Read the model definition and answer for the solid it produces. Units are mm, in the model's axes. A direction names the side the tool comes from. Coordinates: 2 decimals unless noted, no trailing zeros. Loops run counter-clockwise (first coordinate to the right, second up) from the corner with the lowest first, then second, coordinate; pieces in that order, holes last.
Q1. Section D-D (z = -81.5) is taken. Give the vertices of the cut face in (x, y).
Q2. Section C-C (y = -30) is taken. Give the vertices of the cut face in (x, z), then the cut area to 3 significant figures.
Q3. The mould has two halves that part along Y. Classify faces 1 (the face through (0.1, 12.5, -15)), 2 (the face through (0.111, -10.465, 11.056)), 3 (the face through (-0.28, 12.08, -10.12)), 4 (the face through (0, 15, 0)): pulls with the +Y half, pulls with the -Y half, needs draft (parallel to the pull), parting line crosses it, or undercut.
Q4. Which of the six approach directions +Z, -Z, +X, -X, +Y, -Y give full straight-line access (tool end or side, diameter ignored) to faces 5 (the face through (-2.938, -22, -60)), 6 (the face through (0, -27, 7)), 7 (the face through (0.323, -3.605, -35.525))?
Q5. Section A-A (z = -64.5) is taken. Give the vertices of the cut face in (x, y), then the cut area to 3 significant figures.
Q6. Flat-ended cylindrical pins translate along their axes: P1, Ø13, axis at y = -18, z = -64.5, coming from the +X side; P2, Ø3, axis at x = -6, z = -83, coming from the +Y side; P3, Ø4.5, axis at x = 0, y = -35, coming from the +Z side; P4, Ø9, axis at x = 0, z = -10, coming from the -Y side. Find the tip coordinate at first contact, or state that the pin passes through.
Q7. Straight lines are drawn through the part: line 1 (Y direction, x = -1.45, z = -64.5); line 2 (X direction, y = -36, z = -22); line 3 (Z direction, x = -0.75, y = -28). For each, find the intervals that lie inside material, in ascending order.
Q8. Section B-B (z = 0.5) is taken. Give the vertices of the cut face in (x, y), then the cut area to 3 significant figures.
from build123d import *

# Parameters (mm, degrees)
ESBO_O1_R                                            = 7
RESSALTO_EXTRUS_O1_DEPTH                             = 7.9375
ESCAREADO_PARA_PARAFUSO_DE_M_QUINA_COM_C_D           = 5.5
ESCAREADO_PARA_PARAFUSO_DE_M_QUINA_COM_C_DEPTH       = 30
ESCAREADO_PARA_PARAFUSO_DE_M_QUINA_COM_C_CSINK_D     = 10.4
ESCAREADO_PARA_PARAFUSO_DE_M_QUINA_COM_C_CSINK_ANGLE = 90
ESCAREADO_PARA_PARAFUSO_DE_M_QUINA_COM_C_TIP         = 1.652366702
ESCAREADO_PARA_PARAFUSO_DE_M_QUINA_C_2_D             = 6.6
ESCAREADO_PARA_PARAFUSO_DE_M_QUINA_C_2_DEPTH         = 30
ESCAREADO_PARA_PARAFUSO_DE_M_QUINA_C_2_CSINK_D       = 12.6
ESCAREADO_PARA_PARAFUSO_DE_M_QUINA_C_2_CSINK_ANGLE   = 90
ESCAREADO_PARA_PARAFUSO_DE_M_QUINA_C_2_TIP           = 1.982840043
BROCA_DE_ROSQUEAR_PARA_TARRAXA_DE_M5X0_8_D           = 4.2
BROCA_DE_ROSQUEAR_PARA_TARRAXA_DE_M5X0_8_DEPTH       = 20
BROCA_DE_ROSQUEAR_PARA_TARRAXA_DE_M5X0_8_TIP         = 1.2618073
BROCA_DE_ROSQUEAR_PARA_TARRAXA_DE_M5_2_D             = 4.2
BROCA_DE_ROSQUEAR_PARA_TARRAXA_DE_M5_2_DEPTH         = 20
BROCA_DE_ROSQUEAR_PARA_TARRAXA_DE_M5_2_TIP           = 1.2618073
BROCA_DE_ROSQUEAR_PARA_TARRAXA_DE_M6X1_0_D           = 5
BROCA_DE_ROSQUEAR_PARA_TARRAXA_DE_M6X1_0_DEPTH       = 15
BROCA_DE_ROSQUEAR_PARA_TARRAXA_DE_M6X1_0_TIP         = 1.502151548
ESCAREADO_PARA_SFHCS_M51_AT_2_COUNT                  = 2
ESCAREADO_PARA_SFHCS_M51_AT_2_PITCH                  = 12
ESCAREADO_PARA_SFHCS_M51_AT_3_COUNT                  = 2
ESCAREADO_PARA_SFHCS_M51_AT_3_PITCH                  = 67.209946437
ESCAREADO_PARA_SFHCS_M51_AT_4_COUNT                  = 2
ESCAREADO_PARA_SFHCS_M51_AT_4_PITCH                  = 66.13
SKETCH1_R                                            = 18.5
CUT_EXTRUDE1_DEPTH                                   = 7.55
SKETCH2_R                                            = 5
CUT_EXTRUDE2_DEPTH                                   = 107.175824146
SKETCH3_R                                            = 9.5
CUT_EXTRUDE3_DEPTH                                   = 5
FILLET1_R                                            = 6


with BuildPart() as part:
    # Esboço1 → Ressalto-extrusão1 (new, symmetric)
    with BuildSketch(Plane(origin=(0, 0, 0), x_dir=(0, 0, -1), z_dir=(1, 0, 0))):
        Polygon((15, 15), (-15, 15), (-15, -6.05572809), (-7, -15), (-7, -40), (98, -40), (98, 4), (15, 4), align=None)
        Circle(ESBO_O1_R, mode=Mode.SUBTRACT)
    extrude(amount=RESSALTO_EXTRUS_O1_DEPTH, both=True)

    # Escareado para parafuso de m_quina com c
    with Locations(Plane(origin=(-33.0625, -33.751665499, 15.070399895), x_dir=(1, 0, 0), z_dir=(0, 0, 1))):
        with Locations((-33.0625, 13.751665499), (-33.0625, -1.248334501), (33.0625, -1.248334501), (33.0625, 13.751665499)):
            CounterSinkHole(ESCAREADO_PARA_PARAFUSO_DE_M_QUINA_COM_C_D / 2, ESCAREADO_PARA_PARAFUSO_DE_M_QUINA_COM_C_CSINK_D / 2, depth=ESCAREADO_PARA_PARAFUSO_DE_M_QUINA_COM_C_DEPTH, counter_sink_angle=ESCAREADO_PARA_PARAFUSO_DE_M_QUINA_COM_C_CSINK_ANGLE)
            with Locations((0, 0, -(ESCAREADO_PARA_PARAFUSO_DE_M_QUINA_COM_C_DEPTH + ESCAREADO_PARA_PARAFUSO_DE_M_QUINA_COM_C_TIP / 2))):  # 118° drill point
                Cone(0, ESCAREADO_PARA_PARAFUSO_DE_M_QUINA_COM_C_D / 2, ESCAREADO_PARA_PARAFUSO_DE_M_QUINA_COM_C_TIP, mode=Mode.SUBTRACT)

    # Escareado para parafuso de m_quina c 2
    with Locations(Plane(origin=(-33.0625, -47, -36.460196829), x_dir=(-1, 0, 0), z_dir=(0, -1, 0))):
        with Locations((33.06, 49.586524306), (33.06, -3.413475694), (-33.06, -3.413475694), (-33.06, 53.539803171)):
            CounterSinkHole(ESCAREADO_PARA_PARAFUSO_DE_M_QUINA_C_2_D / 2, ESCAREADO_PARA_PARAFUSO_DE_M_QUINA_C_2_CSINK_D / 2, depth=ESCAREADO_PARA_PARAFUSO_DE_M_QUINA_C_2_DEPTH, counter_sink_angle=ESCAREADO_PARA_PARAFUSO_DE_M_QUINA_C_2_CSINK_ANGLE)
            with Locations((0, 0, -(ESCAREADO_PARA_PARAFUSO_DE_M_QUINA_C_2_DEPTH + ESCAREADO_PARA_PARAFUSO_DE_M_QUINA_C_2_TIP / 2))):  # 118° drill point
                Cone(0, ESCAREADO_PARA_PARAFUSO_DE_M_QUINA_C_2_D / 2, ESCAREADO_PARA_PARAFUSO_DE_M_QUINA_C_2_TIP, mode=Mode.SUBTRACT)

    # Broca de rosquear para tarraxa de M5x0.8
    with Locations(Plane(origin=(-33.0625, 25, -36.460196829), x_dir=(1, 0, 0), z_dir=(0, 1, 0))):
        with Locations((33.06, -45.460196829), (-33.065, -45.460196829)):
            Hole(BROCA_DE_ROSQUEAR_PARA_TARRAXA_DE_M5X0_8_D / 2, depth=BROCA_DE_ROSQUEAR_PARA_TARRAXA_DE_M5X0_8_DEPTH)
            with Locations((0, 0, -(BROCA_DE_ROSQUEAR_PARA_TARRAXA_DE_M5X0_8_DEPTH + BROCA_DE_ROSQUEAR_PARA_TARRAXA_DE_M5X0_8_TIP / 2))):  # 118° drill point
                Cone(0, BROCA_DE_ROSQUEAR_PARA_TARRAXA_DE_M5X0_8_D / 2, BROCA_DE_ROSQUEAR_PARA_TARRAXA_DE_M5X0_8_TIP, mode=Mode.SUBTRACT)

    # Broca de rosquear para tarraxa de M5 2
    with Locations(Plane(origin=(-33.0625, -33.751665499, -25), x_dir=(-1, 0, 0), z_dir=(0, 0, -1))):
        with Locations((-33.06, 43.751665499), (33.065, 43.751665499)):
            Hole(BROCA_DE_ROSQUEAR_PARA_TARRAXA_DE_M5_2_D / 2, depth=BROCA_DE_ROSQUEAR_PARA_TARRAXA_DE_M5_2_DEPTH)
            with Locations((0, 0, -(BROCA_DE_ROSQUEAR_PARA_TARRAXA_DE_M5_2_DEPTH + BROCA_DE_ROSQUEAR_PARA_TARRAXA_DE_M5_2_TIP / 2))):  # 118° drill point
                Cone(0, BROCA_DE_ROSQUEAR_PARA_TARRAXA_DE_M5_2_D / 2, BROCA_DE_ROSQUEAR_PARA_TARRAXA_DE_M5_2_TIP, mode=Mode.SUBTRACT)

    # Broca de rosquear para tarraxa de M6x1.01
    with Locations(Plane(origin=(-33.0625, 4, -36.460196829), x_dir=(1, 0, 0), z_dir=(0, 1, 0))):
        with Locations((33.06, 53.539803171), (-33.06, 49.539803171), (-33.06, -3.413475694), (33.06, -3.413475694)):
            Hole(BROCA_DE_ROSQUEAR_PARA_TARRAXA_DE_M6X1_0_D / 2, depth=BROCA_DE_ROSQUEAR_PARA_TARRAXA_DE_M6X1_0_DEPTH)
            with Locations((0, 0, -(BROCA_DE_ROSQUEAR_PARA_TARRAXA_DE_M6X1_0_DEPTH + BROCA_DE_ROSQUEAR_PARA_TARRAXA_DE_M6X1_0_TIP / 2))):  # 118° drill point
                Cone(0, BROCA_DE_ROSQUEAR_PARA_TARRAXA_DE_M6X1_0_D / 2, BROCA_DE_ROSQUEAR_PARA_TARRAXA_DE_M6X1_0_TIP, mode=Mode.SUBTRACT)

    # Esboço23 → Escareado para SFHCS M51 (revolve, cut)
    with BuildSketch(Plane(origin=(0.0025, -57, -22), x_dir=(0, 0, -1), z_dir=(1, 0, 0))):
        Polygon((0, 0), (0, 31.652366702), (2.75, 30), (2.75, 3.35), (5.6, 0.5), (5.6, 0), align=None)
    escareado_para_sfhcs_m51 = revolve(axis=Axis((0.0025, -63.35, -22), (0, 1, 0)), mode=Mode.SUBTRACT)

    # Escareado para SFHCS M51 at 2: Escareado para SFHCS M51 ×2
    with Locations(*[(0, 0, i * ESCAREADO_PARA_SFHCS_M51_AT_2_PITCH) for i in range(1, ESCAREADO_PARA_SFHCS_M51_AT_2_COUNT)]):
        add(escareado_para_sfhcs_m51, mode=Mode.SUBTRACT)

    # Escareado para SFHCS M51 at 3: Escareado para SFHCS M51 ×2
    with Locations(*[Vector(-0.9839317468056482, 0, 0.17854500168861012) * (i * ESCAREADO_PARA_SFHCS_M51_AT_3_PITCH) for i in range(1, ESCAREADO_PARA_SFHCS_M51_AT_3_COUNT)]):
        add(escareado_para_sfhcs_m51, mode=Mode.SUBTRACT)

    # Escareado para SFHCS M51 at 4: Escareado para SFHCS M51 ×2
    with Locations(*[(-i * ESCAREADO_PARA_SFHCS_M51_AT_4_PITCH, 0, 0) for i in range(1, ESCAREADO_PARA_SFHCS_M51_AT_4_COUNT)]):
        add(escareado_para_sfhcs_m51, mode=Mode.SUBTRACT)

    # Sketch1 → Cut-Extrude1 (cut)
    with BuildSketch(Plane(origin=(7.9375, 0, 0), x_dir=(0, 0, -1), z_dir=(1, 0, 0))):
        with Locations((64.5, -18)):
            Circle(SKETCH1_R)
    extrude(amount=-CUT_EXTRUDE1_DEPTH, mode=Mode.SUBTRACT)

    # Sketch2 → Cut-Extrude2 (cut, through all)
    with BuildSketch(Plane(origin=(0.3875, 0, 0), x_dir=(0, 0, -1), z_dir=(1, 0, 0))):
        with Locations((64.5, -18)):
            Circle(SKETCH2_R)
    extrude(amount=-CUT_EXTRUDE2_DEPTH, mode=Mode.SUBTRACT)

    # Sketch3 → Cut-Extrude3 (cut)
    with BuildSketch(Plane.ZY.offset(7.9375)):
        with Locations((-64.5, -18)):
            Circle(SKETCH3_R)
    extrude(amount=-CUT_EXTRUDE3_DEPTH, mode=Mode.SUBTRACT)

    # Fillet1
    # the kernel refuses this fillet: 6 mm, written as the material it adds along each edge
    with BuildSketch(Plane(origin=(7.9375, 4, -15), x_dir=(0, 1, 0), z_dir=(-1, 0, 0))) as fillet1_piece_1_section:
        with BuildLine():
            CenterArc((FILLET1_R, FILLET1_R), FILLET1_R, 180, 90)
            Line((0, FILLET1_R), (0, 0))
            Line((0, 0), (FILLET1_R, 0))
        make_face()
    fillet1_piece_1 = extrude(amount=15.875, mode=Mode.PRIVATE)
    fillet1_piece_1 = fillet1_piece_1 - Plane(origin=(-0.0025, 10, -16.372210647), x_dir=(1, 0, 0), z_dir=(0, 0, 1)) * Cylinder(2.1, 56, mode=Mode.PRIVATE)
    add(fillet1_piece_1)


solid = part.part
Numbers:
1. outline: (-7.94, -40) - (7.94, -40) - (7.94, -25.3) - (0.39, -25.3) - (0.39, -10.7) - (7.94, -10.7) - (7.94, 4) - (-7.94, 4) - close
2. outline: (-7.94, -98) - (7.94, -98) - (7.94, -78.58) - (0.39, -78.58) - (0.39, -50.42) - (7.94, -50.42) - (7.94, 7) - (-7.94, 7) - close; hole circle Ø6.6 at (0, -90); hole circle Ø6.6 at (0, -33.05); hole circle Ø5.5 at (0, -22); hole circle Ø5.5 at (0, -10)
2. area: 1,340 mm2
3. face 1: needs draft
3. face 2: pulls with the -Y half
3. face 3: undercut
3. face 4: pulls with the +Y half
4. face 5: -X
4. face 6: +Z, +X, -X, -Y
4. face 7: +Y
5. outline: (-7.94, -40) - (7.94, -40) - (7.94, -36.5) - (0.39, -36.5) - (0.39, -23) - (-2.94, -23) - (-2.94, -27.5) - (-7.94, -27.5) - close; (-7.94, -8.5) - (-2.94, -8.5) - (-2.94, -13) - (0.39, -13) - (0.39, 0.5) - (7.94, 0.5) - (7.94, 4) - (-7.94, 4) - close
5. area: 291 mm2
6. P1: stops at x = 0.39
6. P2: stops at y = 4
6. P3: stops at z = -15.23
6. P4: stops at y = -40
7. line 1: y = -40 to -23, -13 to 4
7. line 2: x = -7.94 to -2.75, 2.75 to 7.94
7. line 3: z = -98 to -93.21, -86.79 to -36.26, -29.83 to -24.65, -19.35 to -12.65, -7.35 to 7
8. outline: (-7.94, -40) - (7.94, -40) - (7.94, -6.98) - (-7.94, -6.98) - close; (-7.94, 6.98) - (7.94, 6.98) - (7.94, 15) - (-7.94, 15) - close; hole circle Ø5.5 at (0, -35); hole circle Ø5.5 at (0, -20)
8. area: 604 mm2
